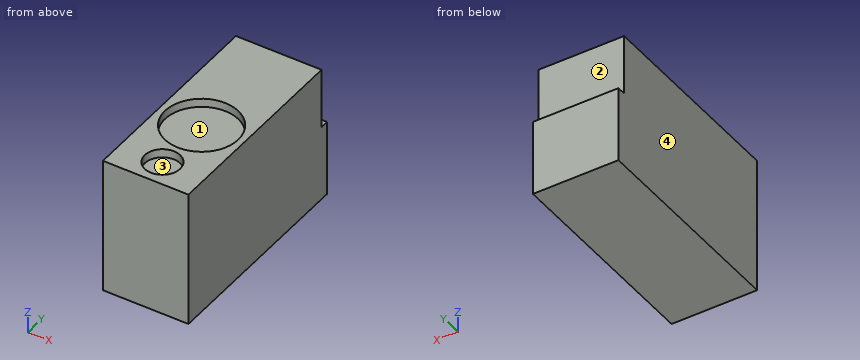
from build123d import *

# Parameters (mm, degrees)
F0_W     = 252.222
F0_H     = 403.352
F1_DEPTH = 629.92
F2_R     = 52.07
F2_R_2   = 107.95
F3_DEPTH = 25.4
F5_W     = 252.222
F5_H     = 25.4
F6_DEPTH = 178.816


with BuildPart() as f1:
    # F0 (on Front) → F1 (new body)
    with BuildSketch(Plane.XZ):
        with Locations((126.111, 201.676)):
            Rectangle(F0_W, F0_H)
    extrude(amount=F1_DEPTH)

    # F2 (on face) → F3 (cut)
    with BuildSketch(Plane.XY.offset(403.352)):
        with Locations((126.111, -553.72)):
            Circle(F2_R)
        with Locations((126.111, -375.92)):
            Circle(F2_R_2)
    extrude(amount=-F3_DEPTH, mode=Mode.SUBTRACT)

    # F5 (on face) → F6 (cut)
    with BuildSketch(Plane.XY.offset(403.352)):
        with Locations((126.111, -12.7)):
            Rectangle(F5_W, F5_H)
    extrude(amount=-F6_DEPTH, mode=Mode.SUBTRACT)


solid = f1.part
Can you work these out from the model? Positions are in its coordinate system, mm. Face numbers are marked on the shaded views. Give positions to 0.01 mm unless a question says otherwise; leave off trailing zeros. Loops run counter-clockwise (first coordinate to the right, second up) from the corner with the lowest first, then second, coordinate; pieces in that order, holes last. Notation, with made-up numbers: (-36, -16) - (23, -16) arc R11 ccw to (23, -3) - close; hole circle Ø11 at (-3, -25.75). An arc over 180 degrees is marked (long way). Return JSON: item names as keys, results as strings.
1. If I drill on line 1 (X direction, y = -553, z = 396); line 2 (Y direction, x = 46, z = 305); line 3 (Z direction, x = 163, y = -386), over which ranges is the centre line in solid material (lowest first)?
Output values:
{"line 1": "x = 0 to 74.05, 178.18 to 252.22", "line 2": "y = -629.92 to -25.4", "line 3": "z = 0 to 377.95"}
2. I want a section at A-A on y = -553.72. Please give me the cut outline in (x, z).
Output values:
{"outline": "(0, 0) - (252.22, 0) - (252.22, 403.35) - (178.18, 403.35) - (178.18, 377.95) - (74.04, 377.95) - (74.04, 403.35) - (0, 403.35) - close"}
3. I'm going to push flat-ended pins straight in: pin 1 Ø5 at (x, z) = (170, 323) entering from +Y; pin 2 Ø7.5 at (x, y) = (156, -16) entering from +Z; pin 3 Ø1 at (x, y) = (121, -449) entering from +Z. Where does each tip first touch, or does it pass through?
Output values:
{"pin 1": "stops at y = -25.4", "pin 2": "stops at z = 224.54", "pin 3": "stops at z = 377.95"}
4. I want a section at B-B on x = 118. Please give me the cut outline in (y, z), and give its area (3 significant figures).
Output values:
{"outline": "(-629.92, 0) - (0, 0) - (0, 224.54) - (-25.4, 224.54) - (-25.4, 403.35) - (-268.28, 403.35) - (-268.28, 377.95) - (-483.56, 377.95) - (-483.56, 403.35) - (-502.29, 403.35) - (-502.29, 377.95) - (-605.15, 377.95) - (-605.15, 403.35) - (-629.92, 403.35) - close", "area": "241,000 mm²"}
5. We'd pull the mould along Y, two halves only. Please class the marked faces 1, 2, 3 and 4: +Y half, -Y half, draft (parallel to the pull), parting line (faces both ways), or undercut.
Output values:
{"face 1": "undercut", "face 2": "+Y half", "face 3": "undercut", "face 4": "draft"}
6. I want a section at D-D on y = -375.92. Please give me the cut outline in (x, z), and give its area (3 significant figures).
Output values:
{"outline": "(0, 0) - (252.22, 0) - (252.22, 403.35) - (234.06, 403.35) - (234.06, 377.95) - (18.16, 377.95) - (18.16, 403.35) - (0, 403.35) - close", "area": "96,300 mm²"}
7. I want a section at C-C on z = 304.5. Please give me the cut outline in (x, y).
Output values:
{"outline": "(0, -629.92) - (252.22, -629.92) - (252.22, -25.4) - (0, -25.4) - close"}
